Study the drawing (mm; zero at the part's minimum x, y, z) and answer. Round coordinates to 2 decimals unless told otherwise and drop trailing zeros. Loops run counter-clockwise (first coordinate to the right, second up) from the corner with the lowest first, then second, coordinate; pieces in that order, holes last. Notation, with made-up numbers: (50, 48.5) - (100, 48.5) arc R23 cw to (100, 84.5) - close; hole circle Ø9 at (79, 61). An arc over 180 degrees is marked (long way). One line per item, written item: value.
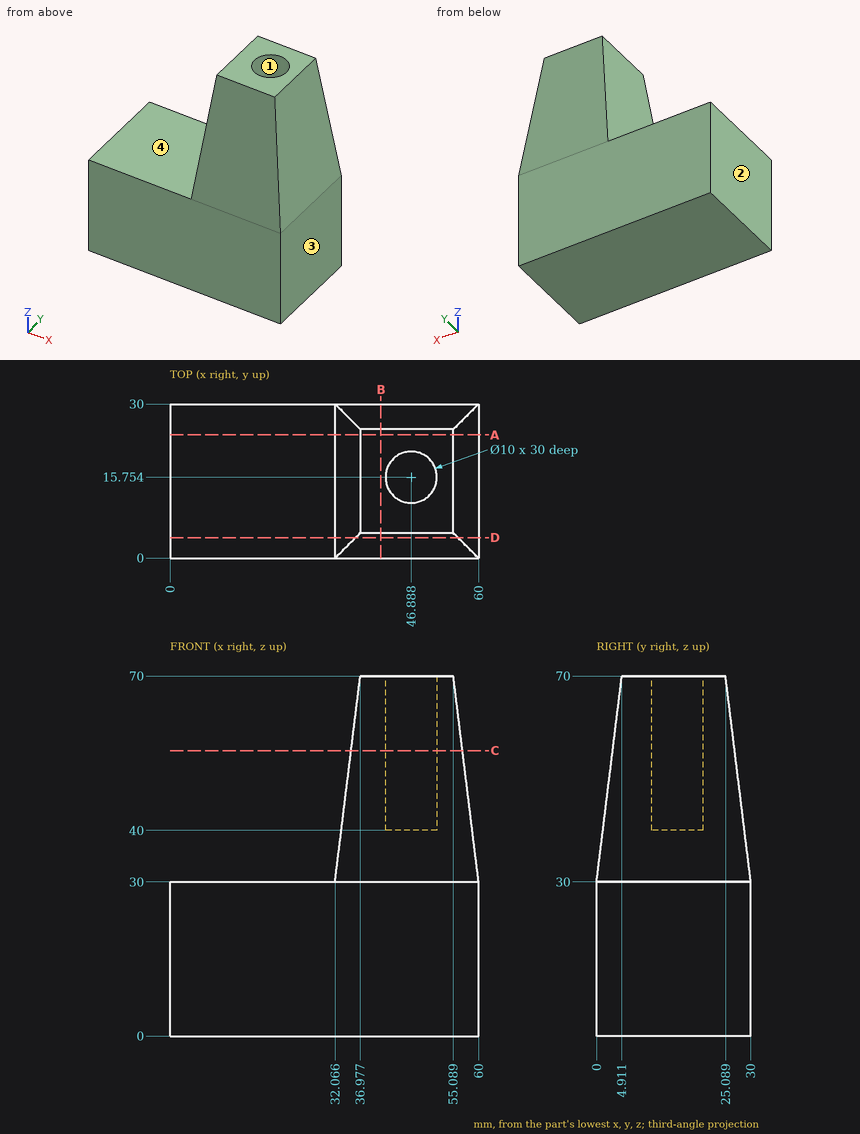
1) A cutting plane is placed at C-C on z = 55.5. Give the vertices of the cut face in (x, y), and give its area (3 significant figures).
Final values:
outline: (35.2, 3.13) - (56.87, 3.13) - (56.87, 26.87) - (35.2, 26.87) - close; hole circle Ø10 at (46.89, 15.75)
area: 436 mm2
2) For a pull along X with two mould halves and no side action, classify the marked faces 1, 2, 3 and 4 as released by +X, released by -X, zero draft, split by the parting line, or undercut.
Final values:
face 1: undercut
face 2: released by -X
face 3: released by +X
face 4: zero draft
3) A cutting plane is placed at A-A on y = 24. Give the vertices of the cut face in (x, z) (1 decimal).
Final values:
outline: (0, 0) - (60, 0) - (60, 30) - (55.1, 70) - (37, 70) - (32.1, 30) - (0, 30) - close
4) A cutting plane is placed at B-B on x = 41. Give the vertices of the cut face in (y, z).
Final values:
outline: (0, 0) - (30, 0) - (30, 30) - (25.09, 70) - (4.91, 70) - (0, 30) - close
5) Each of these flat-tipped pins is pushed along its axis until it touches: pin 1 Ø5 at (y, z) = (18.5, 33) entering from -X; pin 2 Ø8 at (x, y) = (47, 16.5) entering from +Z; pin 3 Ø4 at (y, z) = (9, 50.5) entering from +X. Where does it stop, or does it pass through?
Final values:
pin 1: x = 32.13
pin 2: z = 40
pin 3: x = 57.73
6) A cutting plane is placed at D-D on y = 4. Give the vertices of the cut face in (x, z) (1 decimal), and give its area (3 significant figures).
Final values:
outline: (0, 0) - (60, 0) - (60, 30) - (56, 62.6) - (36.1, 62.6) - (32.1, 30) - (0, 30) - close
area: 2,580 mm2
7) Consider L1, parallel to Z at x = 13.5, y = 4; L2, parallel to X at y = 13.25, z = 48.5 (1 decimal); L3, parallel to X at y = 22.75, z = 45. Determine where each line is inside the solid, lowest interval first.
Final values:
L1: 0 to 30
L2: 34.3 to 42.6, 51.2 to 57.7
L3: 33.91 to 58.16
